CAD build for the part. Positions are in the model's coordinates, mm. A direction names the side the tool comes from. Round coordinates to 2 decimals unless told otherwise and drop trailing zeros. Loops run counter-clockwise (first coordinate to the right, second up) from the corner with the lowest first, then second, coordinate; pieces in that order, holes last. Notation, with made-up numbers: (64, -26) - (82, -26) arc R18 cw to (82, -18) - close; hole circle Ø5 at (72, 68). An arc over 180 degrees is marked (long way). One line per question, with ' | ' between items.
```python
from build123d import *

# Parameters (mm, degrees)
F0_R        = 40.0443714264
F1_DEPTH    = 80
F2_R        = 25.0697968859
F3_DEPTH    = 70
F4_S5_R     = 25.0697968859
F4_T6_DEPTH = 59
F5_R        = 5
F6_R        = 5
F7_T        = -2


# Not quite as in the source:
# - a fillet or chamfer that OpenCascade refuses, or shapes differently, is made with other operations: its cross-section is extruded or revolved along the edge and cut away or added


with BuildPart() as f1:
    # F0 (on Front) → F1 (new body)
    with BuildSketch(Plane.XZ):
        Circle(F0_R)
    extrude(amount=-F1_DEPTH)

    # F2 (on face) → F3 (join)
    with BuildSketch(Plane(origin=(0, 80, 0), x_dir=(-1, 0, 0), z_dir=(0, 1, 0))):
        Circle(F2_R)
    extrude(amount=F3_DEPTH)

    # F4: chamfer of 15 on 1 edges, made by hand


with BuildPart() as f4_tool2:
    # F4_s3 → F4_t4 (revolve)
    with BuildSketch(Plane.XY):
        Polygon((40.0443714264, 65), (25.0443714264, 80), (40.0443714264, 80), align=None)
    revolve(axis=Axis((0, 80, 0), (0, -1, 0)))

    # F4_s5 → F4_t6 (cut, symmetric)
    with BuildSketch(Plane.XZ.offset(-72.5)):
        Circle(F4_S5_R)
    extrude(amount=F4_T6_DEPTH, both=True, mode=Mode.SUBTRACT)


with BuildPart() as f1_1:
    add(f1.part)

    # F4_t1: cut F4_tool2
    add(f4_tool2.part, mode=Mode.SUBTRACT)

    # F5
    f5_edges = [f1_1.edges().sort_by_distance(p)[0] for p in [
        (25.069797, 150, 0),
    ]]
    fillet(f5_edges, radius=F5_R)

    # F6
    f6_edges = [f1_1.edges().sort_by_distance(p)[0] for p in [
        (32.557084, 72.487287, 0),
        (-25.069797, 79.974575, 0),
        (-40.044371, 65, 0),
    ]]
    fillet(f6_edges, radius=F6_R)

    # F7
    f7_openings = [f1_1.faces().sort_by_distance(p)[0] for p in [
        (0, 0, 0),
    ]]
    offset(amount=F7_T, openings=f7_openings)


solid = f1_1.part
```
(1) Cut at B-B, the plane y = 11. Write the cut outline in (x, z).
Results found:
outline: circle Ø80.09 at (0, 0); hole circle Ø76.09 at (0, 0)
(2) Drop flat-ended pins along their axis: P1, Ø5, axis at x = 26.5, y = 22, coming from the -Z side; P2, Ø8, axis at y = 78.5, z = 17.5, coming from the +X side; P3, Ø12, axis at x = 6, z = 2.5, coming from the -Y side. Give the stop position or say it passes through.
Results found:
P1: stops at z = -32.06 | P2: stops at x = 25.7 | P3: stops at y = 148
(3) Cut at A-A, the plane y = 87. Write the cut outline in (x, z), then the cut area to 3 significant figures.
Results found:
outline: circle Ø50.14 at (0, 0); hole circle Ø46.14 at (0, 0) | area: 302 mm²
(4) Two-plate mould, pull along X, no slides. Class faces 4 (the face through (0, 150, 0)), 5 (the face through (36.288, 31.024, 11.427)), 6 (the face through (36.99, 31.02, -15.34)), 7 (the face through (18.307, 113.082, -14.038)): released by +X, released by -X, zero draft, split by the parting line, or undercut.
Results found:
face 4: zero draft | face 5: undercut | face 6: split by the parting line | face 7: undercut
(5) Probe L1, parallel to Z at x = 0, y = 105; L2, parallel to X at y = 35, z = 0. List the from-to ranges inside material, lowest first.
Results found:
L1: z = -25.07 to -23.07, 23.07 to 25.07 | L2: x = -40.04 to -38.04, 38.04 to 40.04
(6) Tool access for faces 1 (the face through (5.435, 113.082, -24.474)), 2 (the face through (14.6, 0, -35.4)), 3 (the face through (0, 148, 0)): list every direction of +Z, -Z, +X, -X, +Y, -Y with a clear straight run to the whole face (end or side of a thin tool).
Results found:
face 1: +Y | face 2: +Z, -Z, +X, -X, -Y | face 3: -Y
